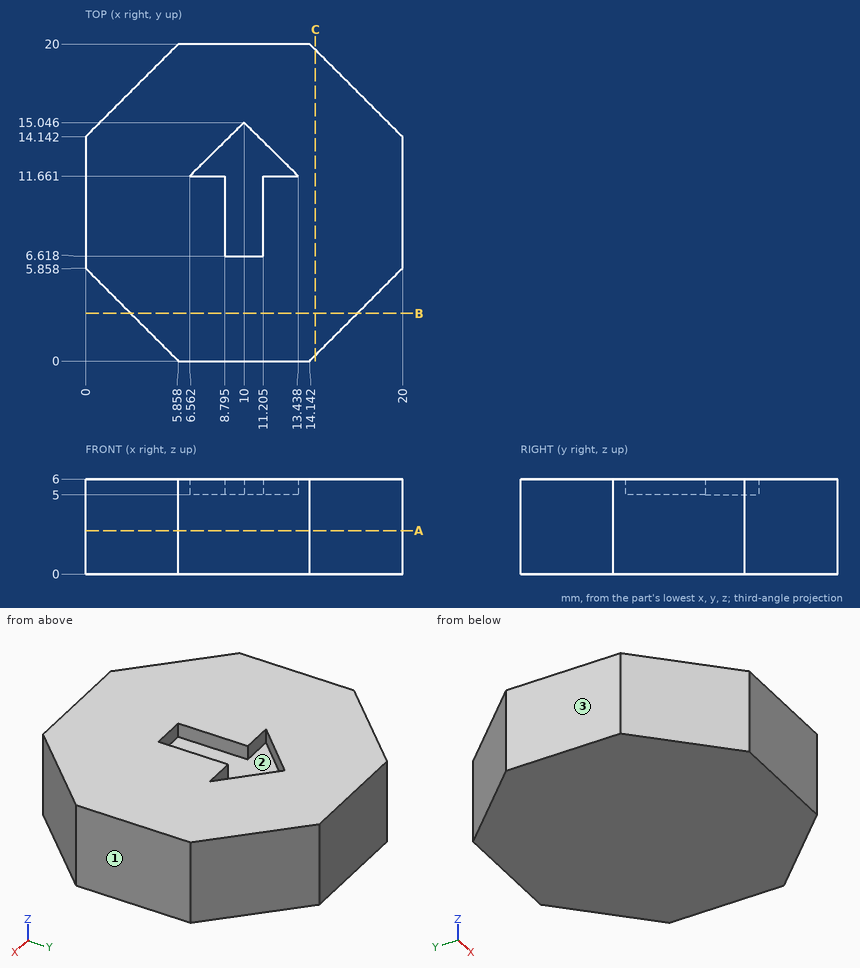
Print and shaded views of the part. All mm, measured from the part's lowest x, y and z. Round coordinates to 2 decimals unless told otherwise and drop trailing zeros. Order: outer loops, then holes, each group sorted by start corner. A loop starts at its lowest first (then second) coordinate and runs counter-clockwise, first axis right, second up.
Q1. Slice it at B-B (y = 3). Write the cut outline in (x, z), and give its area (3 significant figures).
Q2. Drop a flat-ended pin along its axis: pin 1 (2 mm diameter, centred on x = 3.5, z = 1, fed in from -Y). Give the stop position or say it passes through.
Q3. Slice it at C-C (x = 14.5). Write the cut outline in (y, z).
Q4. Wall check: L1, parallel to X at y = 11.25, z = 5.05 (1 decimal); L2, parallel to Z at x = 10.25, y = 12; L3, parallel to Y at x = 5, z = 1.45. Give the ranges that are in metal, low to high.
Q5. Two-plate mould, pull along X, no slides. Class the marked faces 1, 2 and 3: pulls with the +X half, pulls with the -X half, needs draft (parallel to the pull), parting line crosses it, or undercut.
Q6. Slice it at A-A (z = 2.75). Write the cut outline in (x, y), and give its area (3 significant figures).
Results below:
1. outline: (2.86, 0) - (17.14, 0) - (17.14, 6) - (2.86, 6) - close
1. area: 85.7 mm2
2. pin 1: stops at y = 1.36
3. outline: (0.36, 0) - (19.64, 0) - (19.64, 6) - (0.36, 6) - close
4. L1: x = 0 to 8.8, 11.2 to 20
4. L2: z = 0 to 5
4. L3: y = 0.86 to 19.14
5. face 1: pulls with the +X half
5. face 2: undercut
5. face 3: pulls with the -X half
6. outline: (0, 5.86) - (5.86, 0) - (14.14, 0) - (20, 5.86) - (20, 14.14) - (14.14, 20) - (5.86, 20) - (0, 14.14) - close
6. area: 331 mm2
